Source: CAD feature listing. Evaluate the final solid. Frame: model axes, mm. A direction names the side the tool comes from. Round coordinates to 2 decimals unless told otherwise and drop trailing zeros. Loops run counter-clockwise (first coordinate to the right, second up) from the corner with the lowest first, then second, coordinate; pieces in that order, holes last. Notation, with made-up numbers: (88.5, 7.25) -> (94.5, 7.25) arc R8 cw to (94.5, 11.25) -> close; hole circle Ø4 at (-15.75, -6). An arc over 180 degrees is marked (long way). Put each result on its own line as item: value. Start each with the question number.
1. Draft query along Y for faces 4 (the flat face through (4, -2, 0)), 5 (the cylindrical face through (3.3, 14.3, 0.6)), 6 (the flat face through (6, 0, 0)), 7 (the cylindrical face through (8.3, 9.2, 0)). Return one class per face: pulls with the +Y half, pulls with the -Y half, needs draft (parallel to the pull), parting line crosses it, or undercut.
2. Cut plane A-A (y = 2.25). Return the cut outline in (x, z).
3. Contact query for flat-ended pins moving along their axis: pin 1 (0.8 mm diameter, centred on y = -1, z = 0, fed in from -X); pin 2 (1.5 mm diameter, centred on x = 1, y = 7.5, fed in from -Z); pin 3 (1 mm diameter, centred on x = 2.5, y = -1, fed in from -Z); pin 4 (4 mm diameter, centred on x = 3, y = 16, fed in from +Z). Output: stop coordinate, or through.
4. Set-up query: faces 1 (the cylindrical face through (5.4, 0.3, 0.3)), 2 (the cylindrical face through (-0.323, 13.36, -0.506)), 3 (the flat face through (-0.5, -1, 0)). Return all of +Z, -Z, +X, -X, +Y, -Y with unobstructed straight access to the full face (end or side cutting, diameter ignored); none if empty.
5. Material intervals for L1, parallel to X at y = 9, z = 0; L2, parallel to Y at x = 8, z = -0.75; L3, parallel to Z at x = 1, y = -0.25, sorted ascending.
```python
from build123d import *

# Parameters (mm, degrees)
FILLET2_R           = 0.6
FILLET3_R           = 0.6
FILLET4_R           = 0.6
FILLET5_R           = 0.6
SKETCH14_W          = 8.5
SKETCH14_H          = 1
BOSS_EXTRUDE1_DEPTH = 2


with BuildPart() as part:
    # Sketch10 → Revolve1 (revolve)
    with BuildSketch(Plane.XY):
        Polygon((0, 0), (-0.5, 0), (-0.5, 0.5), (-0.8, 0.5), (-0.8, 12.15), (-1, 12.15), (-1, 12.65), (-0.6, 12.65), (-0.6, 14.65), (0, 14.65), align=None)
    revolve(axis=Axis((0, 14.65, 0), (0, -1, 0)))

    # Fillet2
    fillet2_edges = [part.edges().sort_by_distance(p)[0] for p in [
        (0.6, 14.65, 0),
    ]]
    fillet(fillet2_edges, radius=FILLET2_R)



with BuildPart() as body_2:
    # Sketch11 → Revolve2 (revolve)
    with BuildSketch(Plane.XY):
        Polygon((2.5, 0), (2, 0), (2, 0.5), (1.7, 0.5), (1.7, 14.01), (1.5, 14.01), (1.5, 14.51), (1.9, 14.51), (1.9, 16.51), (2.5, 16.51), align=None)
    revolve(axis=Axis((2.5, 16.51, 0), (0, -1, 0)))

    # Fillet3
    fillet3_edges = [body_2.edges().sort_by_distance(p)[0] for p in [
        (3.1, 16.51, 0),
    ]]
    fillet(fillet3_edges, radius=FILLET3_R)


with BuildPart() as body_3:
    # Sketch12 → Revolve3 (revolve)
    with BuildSketch(Plane.XY):
        Polygon((5, 0), (4.5, 0), (4.5, 0.5), (4.2, 0.5), (4.2, 15.88), (4, 15.88), (4, 16.38), (4.4, 16.38), (4.4, 18.38), (5, 18.38), align=None)
    revolve(axis=Axis((5, 18.38, 0), (0, -1, 0)))

    # Fillet4
    fillet4_edges = [body_3.edges().sort_by_distance(p)[0] for p in [
        (5.6, 18.38, 0),
    ]]
    fillet(fillet4_edges, radius=FILLET4_R)


with BuildPart() as body_4:
    # Sketch13 → Revolve4 (revolve)
    with BuildSketch(Plane.XY):
        Polygon((7.5, 0), (7, 0), (7, 0.5), (6.7, 0.5), (6.7, 17.65), (6.5, 17.65), (6.5, 18.15), (6.9, 18.15), (6.9, 20.15), (7.5, 20.15), align=None)
    revolve(axis=Axis((7.5, 20.15, 0), (0, -1, 0)))

    # Fillet5
    fillet5_edges = [body_4.edges().sort_by_distance(p)[0] for p in [
        (8.1, 20.15, 0),
    ]]
    fillet(fillet5_edges, radius=FILLET5_R)


with BuildPart() as part_1:
    add(part.part)

    add(body_2.part)  # Boss-Extrude1 merges body 2

    add(body_3.part)  # Boss-Extrude1 merges body 3

    add(body_4.part)  # Boss-Extrude1 merges body 4
    # Sketch14 → Boss-Extrude1 (add)
    with BuildSketch(Plane.XZ):
        with Locations((3.75, 0)):
            Rectangle(SKETCH14_W, SKETCH14_H)
    extrude(amount=BOSS_EXTRUDE1_DEPTH)


solid = part_1.part
```
Solution:
1. face 4: pulls with the -Y half
1. face 5: needs draft
1. face 6: undercut
1. face 7: undercut
2. outline: circle Ø1.6 at (0, 0); circle Ø1.6 at (2.5, 0); circle Ø1.6 at (5, 0); circle Ø1.6 at (7.5, 0)
3. pin 1: stops at x = -0.5
3. pin 2: stops at z = -0.76
3. pin 3: stops at z = -0.5
3. pin 4: stops at z = 1
4. face 1: none
4. face 2: +Y
4. face 3: +Z, -Z, -X, -Y
5. L1: x = -0.8 to 0.8, 1.7 to 3.3, 4.2 to 5.8, 6.7 to 8.3
5. L2: y = 17.65 to 18.15
5. L3: z = -0.5 to 0.5
